Part print with two shaded views. Sizes in mm from the minimum x, y, z corner. Give positions to 0.01 mm unless a question says otherwise; leave off trailing zeros. Write each loop counter-clockwise with the first axis right and the second up, starting at its lowest first coordinate (ties: lowest second). Pieces come first, ordered by that corner, then holes.
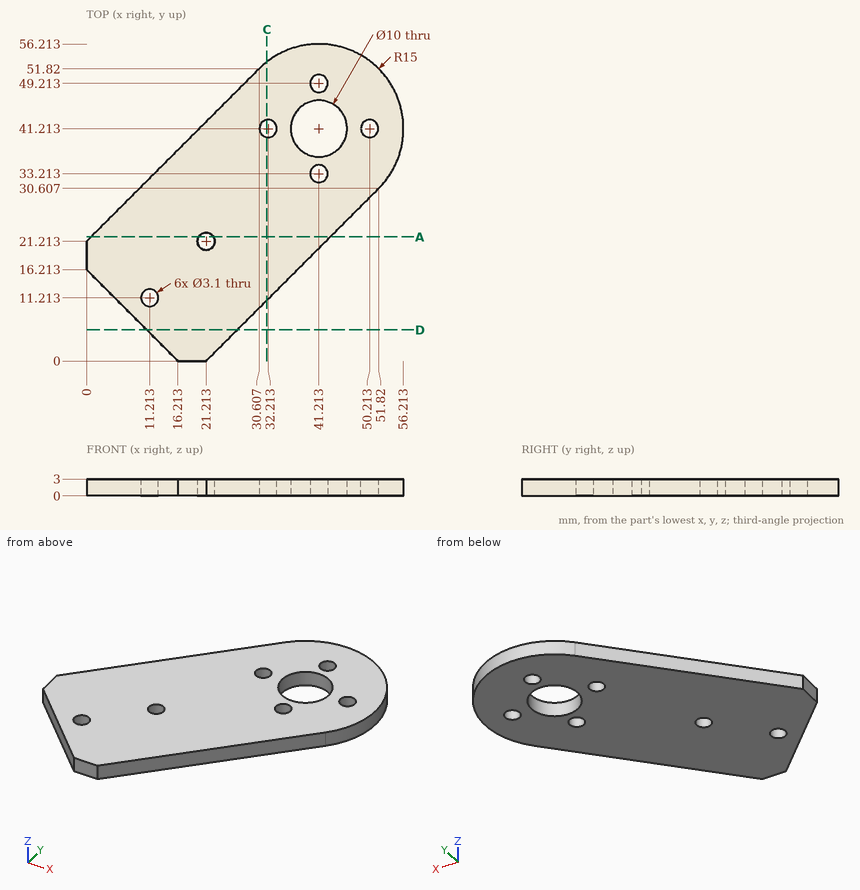
(1) Drop a flat-ended pin along its axis: pin 1 (1 mm diameter, centred on y = 43.5, z = 0.5, fed in from -X). Give the stop position or say it passes through.
(2) Saw through at A-A, the plane y = 22. List the corners of the cut face in (x, z).
(3) Saw through at C-C, the plane x = 32. List the corners of the cut face in (y, z), plus the area to 3 significant figures.
(4) Saw through at D-D, the plane y = 5.5. List the corners of the cut face in (x, z).
(5) Probe line 1 (X direction, y = 39.5, z = 1.3) (1 decimal); line 2 (X direction, y = 6.5, z = 1.4) (1 decimal); line 3 (X direction, y = 33.5, z = 1.3) (1 decimal). List the from-to ranges inside material, lowest first.
Computed values:
1. pin 1: stops at x = 21.79
2. outline: (0.79, 0) - (19.88, 0) - (19.88, 3) - (0.79, 3) - close; (22.55, 0) - (43.21, 0) - (43.21, 3) - (22.55, 3) - close
3. outline: (10.79, 0) - (39.68, 0) - (39.68, 3) - (10.79, 3) - close; (42.75, 0) - (53.05, 0) - (53.05, 3) - (42.75, 3) - close
3. area: 118 mm2
4. outline: (10.71, 0) - (26.71, 0) - (26.71, 3) - (10.71, 3) - close
5. line 1: x = 18.3 to 36.5, 45.9 to 56.1
5. line 2: x = 9.7 to 27.7
5. line 3: x = 12.3 to 39.7, 42.7 to 54.1
